Autodesk Inventor part; units mm, degrees
ref_plane "YZ Plane" through (0, 0, 0) normal (1, 0, 0) x (0, 1, 0)
ref_plane "XZ Plane" through (0, 0, 0) normal (0, 1, 0) x (-1, 0, 0)
ref_plane "XY Plane" through (0, 0, 0) normal (0, 0, 1) x (1, 0, 0)
sketch "スケッチ1" plane through (0, 0, 0) normal (0, 1, 0) x (-1, 0, 0)
  line L0 (39.4, -27.2) -> (0, -27.2)
  line L1 (0, -27.2) -> (0, 27.2)
  line L2 (0, 27.2) -> (39.4, 27.2)
  line L3 (39.4, -16.3) -> (30.9, -16.3)
  line L4 (30.9, -16.3) -> (30.9, 4.7)
  line L5 (30.9, 4.7) -> (39.4, 4.7)
  line L6 (39.4, 4.7) -> (39.4, -16.3) construction
  line L7 (39.4, 27.2) -> (39.4, 4.7)
  line L8 (39.4, -16.3) -> (39.4, -27.2)
  point P0 (0, 0)
  point P1 (0, 0)
  dimension "d0" = 10.9
  dimension "d1" = 22.5
  dimension "d2" = 39.4
  dimension "d3" = 21
  dimension "d5" = 8.5
extrude "押し出し1" add sketch "スケッチ1" along normal blind 1.6
sketch "スケッチ2" plane through (0, 1.6, 0) normal (0, 1, 0) x (1, 0, 0)
  line L0 (-30.9, 16.3) -> (-30.9, -4.7)
  line L1 (-30.9, -4.7) -> (-39.4, -4.7)
  line L2 (-39.4, -4.7) -> (-39.4, -27.2)
  line L3 (-39.4, -27.2) -> (0, -27.2)
  line L4 (0, -27.2) -> (0, 27.2)
  line L5 (0, 27.2) -> (-39.4, 27.2)
  line L6 (-39.4, 27.2) -> (-39.4, 16.3)
  line L7 (-39.4, 16.3) -> (-30.9, 16.3)
  point P0 (0, 0)
  point P1 (-35.9, 21.55)
  point P2 (-35.9, -15.95)
  dimension "d8" = 11.25
  dimension "d9" = 5.25
  dimension "d10" = 3.5
  dimension "d11" = 3.5
hole "穴1" at (-35.9, 1.6, -21.55) at (-35.9, 1.6, 15.95) direction (0, -1, 0) diameter 1.8 end through all
mirror "ミラー1" about plane through (0, 0, 27.2) normal (1, 0, 0) of "押し出し1"
ref_plane "作業平面1" through (0, 0, 4.7) normal (-1, 0, 0) x (0, 0, 1)
mirror "ミラー2" about plane through (0, 0, 4.7) normal (-1, 0, 0) of "穴1", "押し出し1"
sketch "スケッチ3" plane through (0, 1.6, 0) normal (0, 1, 0) x (1, 0, 0)
  circle A0 centre (35.9, 21.55) radius 0.9
  circle A1 centre (35.9, -15.95) radius 0.9
  line L0 (-39.4, 27.2) -> (39.4, 27.2)
  line L1 (-39.4, 27.2) -> (-39.4, 16.3)
  line L2 (-39.4, 16.3) -> (-30.9, 16.3)
  line L3 (-30.9, 16.3) -> (-30.9, -4.7)
  line L4 (-30.9, -4.7) -> (-39.4, -4.7)
  line L5 (-39.4, -4.7) -> (-39.4, -27.2)
  line L6 (-39.4, -27.2) -> (39.4, -27.2)
  line L7 (39.4, -4.7) -> (39.4, -27.2)
  line L8 (30.9, -4.7) -> (39.4, -4.7)
  line L9 (30.9, 16.3) -> (30.9, -4.7)
  line L10 (39.4, 16.3) -> (30.9, 16.3)
  line L11 (39.4, 27.2) -> (39.4, 16.3)
  circle A2 centre (-35.9, 21.55) radius 0.9
  circle A3 centre (-35.9, -15.95) radius 0.9
  line L12 (-15, 22.2) -> (0, 22.2)
  line L13 (0, 22.2) -> (0, 2.2)
  line L14 (0, 2.2) -> (-15, 2.2)
  line L15 (-15, 2.2) -> (-15, 22.2)
  line L16 (15, 22.2) -> (0, 22.2)
  line L17 (0, 2.2) -> (15, 2.2)
  line L18 (15, 2.2) -> (15, 22.2)
  line L19 (-39.4, 16.3) -> (-30.9, 16.3)
  line L20 (-30.9, 16.3) -> (-30.9, -4.7)
  line L21 (30.9, 16.3) -> (30.9, -4.7)
  line L22 (30.9, -4.7) -> (30.9, 16.3)
  line L23 (-30.9, 16.3) -> (-30.9, -4.7)
  point P0 (0, 0)
  point P1 (0, 12.2)
  dimension "d19" = 30
  dimension "d21" = 20
  dimension "d26" = 5
  dimension "d28" = 39.4
extrude "押し出し2" cut sketch "スケッチ3" against normal blind 10 contours L12 L13 L14 L15 | L16 L18 L17 L13
fillet "フィレット1" radius 2.5 4 edges at (-15, 0.8, -22.2) (-15, 0.8, -2.2) (15, 0.8, -2.2) (15, 0.8, -22.2)
equation "\"d17\" = Thickness"
equation "\"BendRadius\" = Thickness"
equation "\"BendReliefWidth\" = Thickness"
equation "\"BendReliefDepth\" = 0.5 * Thickness"
equation "\"CornerReliefSize\" = 4 * Thickness"
equation "\"MinimumRemnant\" = 2 * Thickness"
equation "\"TransitionRadius\" = BendRadius"
equation "\"JacobiRadiusSize\" = BendRadius"
equation "\"GapSize\" = Thickness"
properties part number "old"
The listing builds one solid part. Answer for the finished solid, in the listing's coordinates (mm). A direction names the side the tool comes from. Coordinates: 2 decimals unless noted, no trailing zeros. Order: outer loops, then holes, each group sorted by start corner. A loop starts at its lowest first (then second) coordinate and runs counter-clockwise, first axis right, second up.
Q1. A cutting plane is placed at B-B, the plane z = 15.95. Write down the section's boundary in (x, y), and give its area (3 significant figures).
Q2. A cutting plane is placed at C-C, the plane y = 0.25. Write down the section's boundary in (x, z), and give its area (3 significant figures).
Q3. Consider line 1 (X direction, y = 1.05, z = 15.95); line 2 (Z direction, x = -35.9, y = 0.7); line 3 (X direction, y = 0.6, z = -21.55). Determine where each line is inside the solid, lowest interval first.
Q4. A cutting plane is placed at A-A, the plane x = 1. Write down the section's boundary in (y, z).
Q5. A cutting plane is placed at D-D, the plane x = -35.9. Write down the section's boundary in (y, z), and give its area (3 significant figures).
Q6. For a pull along Z with two mould halves and no side action, classify faces 5 (the face through (35, 1, -16.3)), 6 (the face through (-1, 1, -27.2)), 7 (the face through (39.4, 1, 16)) as pulls with the +Z half, pulls with the -Z half, needs draft (parallel to the pull), parting line crosses it, or undercut.
Q7. Given P1, Ø1.1, axis at x = 35.9, z = 15.95, coming from the -Y side; P2, Ø3, axis at x = 35.9, z = -21.55, coming from the -Y side; P3, Ø0.5, axis at y = 0.5, z = -7, coming from the +X side; P4, Ø0.8, axis at y = 1, z = -13.5, coming from the -X side, each flat-ended and moving along its own axis, determine where each tip first touches the part or whether it passes through.
Q8. Which of the six approach directions +Z, -Z, +X, -X, +Y, -Y give full straight-line access (tool end or side, diameter ignored) to faces 1 (the face through (15, 1, -12)), 2 (the face through (-35, 1, -16.3)), 3 (the face through (30.9, 1, -6)), 4 (the face through (39.4, 1, -22))?
Answers follow:
1. outline: (-39.4, 0) - (-36.8, 0) - (-36.8, 1.6) - (-39.4, 1.6) - close; (-35, 0) - (35, 0) - (35, 1.6) - (-35, 1.6) - close; (36.8, 0) - (39.4, 0) - (39.4, 1.6) - (36.8, 1.6) - close
1. area: 120 mm2
2. outline: (-39.4, -27.2) - (39.4, -27.2) - (39.4, -16.3) - (30.9, -16.3) - (30.9, 4.7) - (39.4, 4.7) - (39.4, 27.2) - (-39.4, 27.2) - (-39.4, 4.7) - (-30.9, 4.7) - (-30.9, -16.3) - (-39.4, -16.3) - close; hole circle Ø1.8 at (-35.9, -21.55); hole circle Ø1.8 at (-35.9, 15.95); hole (-15, -19.7) arc R2.5 ccw to (-12.5, -22.2) - (12.5, -22.2) arc R2.5 ccw to (15, -19.7) - (15, -4.7) arc R2.5 ccw to (12.5, -2.2) - (-12.5, -2.2) arc R2.5 ccw to (-15, -4.7) - close; hole circle Ø1.8 at (35.9, -21.55); hole circle Ø1.8 at (35.9, 15.95)
2. area: 3,320 mm2
3. line 1: x = -39.4 to -36.8, -35 to 35, 36.8 to 39.4
3. line 2: z = -27.2 to -22.45, -20.65 to -16.3, 4.7 to 15.05, 16.85 to 27.2
3. line 3: x = -39.4 to -36.8, -35 to -14.18, 14.18 to 35, 36.8 to 39.4
4. outline: (0, -27.2) - (1.6, -27.2) - (1.6, -22.2) - (0, -22.2) - close; (0, -2.2) - (1.6, -2.2) - (1.6, 27.2) - (0, 27.2) - close
5. outline: (0, -27.2) - (1.6, -27.2) - (1.6, -22.45) - (0, -22.45) - close; (0, -20.65) - (1.6, -20.65) - (1.6, -16.3) - (0, -16.3) - close; (0, 4.7) - (1.6, 4.7) - (1.6, 15.05) - (0, 15.05) - close; (0, 16.85) - (1.6, 16.85) - (1.6, 27.2) - (0, 27.2) - close
5. area: 47.7 mm2
6. face 5: undercut
6. face 6: pulls with the -Z half
6. face 7: needs draft
7. P1: passes through
7. P2: stops at y = 0
7. P3: stops at x = 30.9
7. P4: stops at x = -30.9
8. face 1: +Y, -Y
8. face 2: -X, +Y, -Y
8. face 3: +X, +Y, -Y
8. face 4: +Z, -Z, +X, +Y, -Y
